Geometry check sheet. Reference: the model listing, model coordinates, mm. Give positions to 0.01 mm unless a question says otherwise; leave off trailing zeros. Loops run counter-clockwise (first coordinate to the right, second up) from the corner with the lowest first, then second, coordinate; pieces in that order, holes last. Notation, with made-up numbers: (-26, 36.5) -> (-9, 36.5) arc R19 cw to (-9, 45.5) -> close; hole circle Ø3 at (75.5, 7.25). An arc over 180 degrees is marked (long way). One line per item, written item: value. Start each with the question number.
(1) Sectioned sample at A-A, the plane x = 63. Record the cut outline in (y, z).
(2) Draft check along Y on faces 1 (the face through (-1, -35, 0)), 2 (the face through (25.828, -1.973, 0.035)), 3 (the face through (-75, 0, 0)). Enter one of: pulls with the +Y half, pulls with the -Y half, needs draft (parallel to the pull), parting line crosses it, or undercut.
(3) Sectioned sample at B-B, the plane z = 1.2. Record the cut outline in (x, y), then the cut area to 3 significant figures.
(4) Scan lines: line 1 along Y through (x, z) = (63, 0.65); line 2 along X through (y, z) = (4.5, 2.35); line 3 along X through (y, z) = (3, 0.65). Record each from-to range of solid material in increasing order. Write a range as from..to.
from build123d import *

# Parameters (mm, degrees)
SKETCH1_W           = 150
SKETCH1_H           = 70
BOSS_EXTRUDE1_DEPTH = 2.5
SKETCH2_R           = 4
CUT_EXTRUDE1_DEPTH  = 6


with BuildPart() as part:
    # Sketch1 → Boss-Extrude1 (new body, symmetric)
    with BuildSketch(Plane.XY):
        Rectangle(SKETCH1_W, SKETCH1_H)
    extrude(amount=BOSS_EXTRUDE1_DEPTH, both=True)

    # Sketch2 → Cut-Extrude1 (cut, through all)
    with BuildSketch(Plane.XY.offset(2.5)):
        with Locations((63, 0.85119924)):
            Circle(SKETCH2_R)
        with Locations((29.002241117, 0.460826454)):
            Circle(SKETCH2_R)
        with Locations((-42.995335398, -0.365871995)):
            Circle(SKETCH2_R)
        with Locations((-3.99705162, 0)):
            Circle(SKETCH2_R)
    extrude(amount=-CUT_EXTRUDE1_DEPTH, mode=Mode.SUBTRACT)


solid = part.part
Calculated:
1. outline: (-35, -2.5) -> (-3.15, -2.5) -> (-3.15, 2.5) -> (-35, 2.5) -> close; (4.85, -2.5) -> (35, -2.5) -> (35, 2.5) -> (4.85, 2.5) -> close
2. face 1: pulls with the -Y half
2. face 2: undercut
2. face 3: needs draft
3. outline: (-75, -35) -> (75, -35) -> (75, 35) -> (-75, 35) -> close; hole circle Ø8 at (-43, -0.37); hole circle Ø8 at (-4, 0); hole circle Ø8 at (29, 0.46); hole circle Ø8 at (63, 0.85)
3. area: 10,300 mm2
4. line 1: y = -35..-3.15, 4.85..35
4. line 2: x = -75..61.36, 64.64..75
4. line 3: x = -75..-45.16, -40.83..-6.64, -1.35..25.91, 32.09..59.63, 66.37..75
